Autodesk Inventor part; units mm, degrees
ref_plane "C3_XY" through (133, 0, 0) normal (-1, 0, 0) x (0, 0, -1)
ref_plane "C3_YZ" through (133, 0, 0) normal (0, 0, -1) x (0, -1, 0)
ref_plane "C3_ZX" through (133, 0, 0) normal (0, -1, 0) x (-1, 0, 0)
sketch "Sketch_1" plane through (0, 0, 0) normal (0, 0, 1) x (1, 0, 0)
  line L0 (133, 0) -> (0, 0)
  line L1 (0, 0) -> (0, 3.5)
  line L2 (0, 3.5) -> (0.6062, 4.55)
  line L3 (0.6062, 4.55) -> (132.3938, 4.55)
  line L4 (132.3938, 4.55) -> (133, 3.5)
  line L5 (133, 3.5) -> (133, 0)
  line L6 (133, 0) -> (0, 0)
revolve "Revolution1" add sketch "Sketch_1" angle 360 about axis through (133, 0, 0) along (1, 0, 0)
sketch "Sketch_2" plane through (0, 0, 0) normal (1, 0, 0) x (0, 1, 0)
  line L0 (7, 7) -> (-7, 7)
  line L1 (-7, 7) -> (-7, -7)
  line L2 (-7, -7) -> (7, -7)
  line L3 (7, -7) -> (7, 7)
  line L4 (-2.0207, 3.5) -> (-4.0415, 0)
  line L5 (-4.0415, 0) -> (-2.0207, -3.5)
  line L6 (-2.0207, -3.5) -> (2.0207, -3.5)
  line L7 (2.0207, -3.5) -> (4.0415, 0)
  line L8 (4.0415, 0) -> (2.0207, 3.5)
  line L9 (2.0207, 3.5) -> (-2.0207, 3.5)
extrude "Extrusion1" cut sketch "Sketch_2" along normal blind 133
sketch "Sketch3" plane through (0, 0, 0) normal (-1, 0, 0) x (0, 0, 1)
  point P0 (0, 0)
hole "Hole1" at (0, 0, 0) direction (1, 0, 0) diameter 2.459 depth 8.2901 tip angle 120 countersink diameter 3 countersink angle 90
sketch "Sketch4" plane through (133, 0, 0) normal (1, 0, 0) x (0, 0, -1)
  point P0 (0, 0)
hole "Hole2" at (133, 0, 0) direction (-1, 0, 0) diameter 2.459 depth 8.2901 tip angle 120 countersink diameter 3 countersink angle 90
ref_plane "C3_XY" through (133, 0, 0) normal (-1, 0, 0) x (0, 0, -1)
ref_plane "C3_YZ" through (133, 0, 0) normal (0, 0, -1) x (0, -1, 0)
ref_plane "C3_ZX" through (133, 0, 0) normal (0, -1, 0) x (-1, 0, 0)
properties part number "ABLSBF7-133-M3-N3"
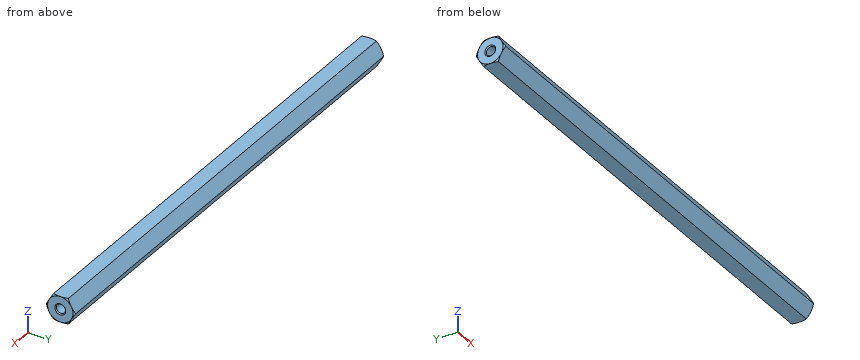
Can you work these out from the model? Positions are in its coordinate system, mm. Coordinates: 2 decimals unless noted, no trailing zeros. Write each loop counter-clockwise with the first axis right and the second up, starting at its lowest first coordinate (ties: lowest second). Pieces come first, ordered by that corner, then holes. Notation, with made-up numbers: (37, 83.5) -> (90, 83.5) arc R9 ccw to (90, 89.5) -> close; hole circle Ø8 at (0, 82). An arc over 180 degrees is marked (long way). Write each question's results on one line, items separated by ' | '. Start each with the question number.
Item 1: If we section it at A-A, the plane x = 75: Write out the boundary of the cut face in (y, z).
Item 2: I'm going to push flat-ended pins straight in: P1, Ø3, axis at x = 34, z = 1, coming from the -Y side; P2, Ø2, axis at y = 0, z = 0, coming from the -X side; P3, Ø1, axis at x = 112, z = -2, coming from the +Y side. Where does each tip first touch, or does it pass through?
Item 3: Please list where these lines run through material, in increasing order: probe 1 along Y at (x, z) = (130.5, 0); probe 2 along Z at (x, y) = (128.75, 0); probe 3 along Y at (x, z) = (104.5, -1.75).
Answer block:
1) outline: (-4.04, 0) -> (-2.02, -3.5) -> (2.02, -3.5) -> (4.04, 0) -> (2.02, 3.5) -> (-2.02, 3.5) -> close
2) P1: y = -4.04 | P2: x = 8.42 | P3: y = 3.18
3) probe 1: -4.04 to -1.23, 1.23 to 4.04 | probe 2: -3.5 to -1.23, 1.23 to 3.5 | probe 3: -3.03 to 3.03
